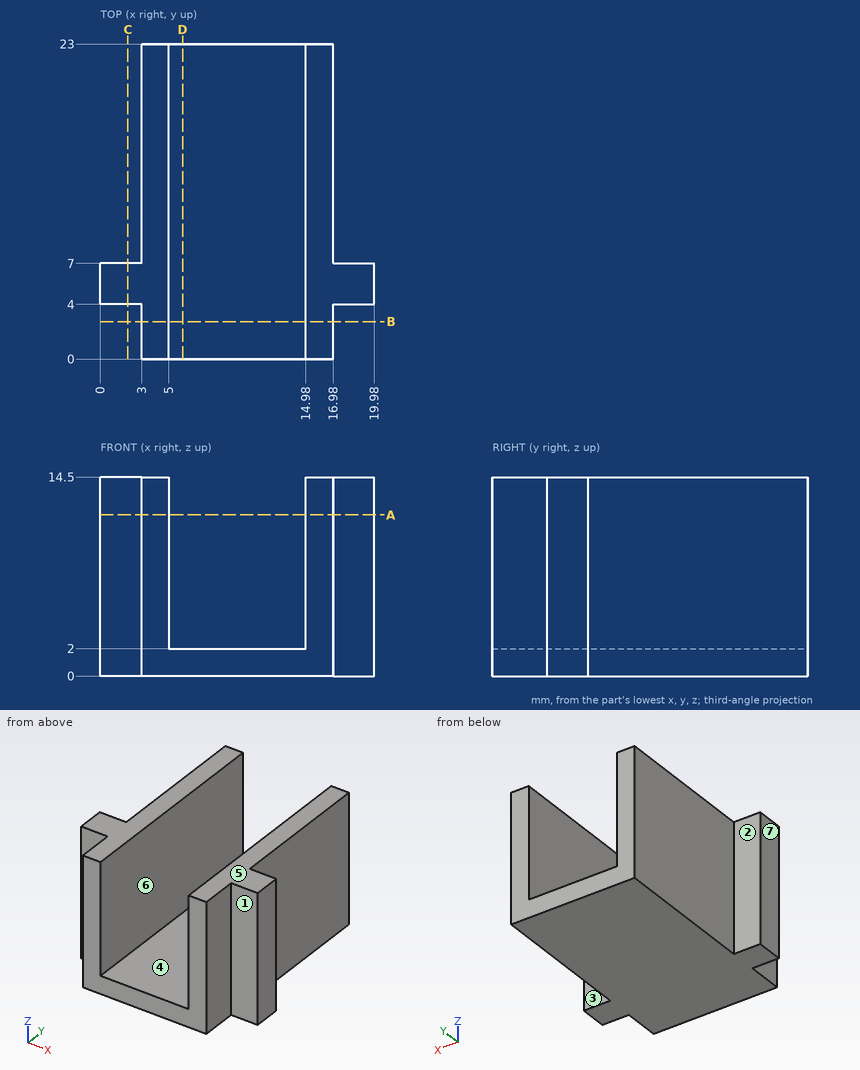
The drawing under review shows one solid part. Ordinate dimensions are in mm from its lowest x, y, z. A direction names the side the tool comes from. Coordinates: 2 decimals unless noted, no trailing zeros. Order: outer loops, then holes, each group sorted by start corner. A loop starts at its lowest first (then second) coordinate and runs counter-clockwise, first axis right, second up. Notation, with made-up numbers: (-4, 27) - (28, 27) arc R23 ccw to (28, 43) - close; hole circle Ø11 at (-34, 48.5). An arc over 180 degrees is marked (long way). Put each result on its own line as item: value.
1) Wall thickness on L1, parallel to X at y = 2.5, z = 9.25; L2, parallel to X at y = 5.5, z = 9; L3, parallel to Z at x = 11.25, y = 13.5: over which ranges is each line inside the solid? List them lowest first. Write a range as from..to.
Response values:
L1: x = 3..5, 14.98..16.98
L2: x = 0..5, 14.98..19.98
L3: z = 0..2
2) Take a section at A-A, the plane z = 11.75. Give the boundary of the cut face in (x, y).
Response values:
outline: (0, 4) - (3, 4) - (3, 0) - (5, 0) - (5, 23) - (3, 23) - (3, 7) - (0, 7) - close; (14.98, 0) - (16.98, 0) - (16.98, 4) - (19.98, 4) - (19.98, 7) - (16.98, 7) - (16.98, 23) - (14.98, 23) - close
3) Take a section at C-C, the plane x = 2. Give the boundary of the cut face in (y, z).
Response values:
outline: (4, 0) - (7, 0) - (7, 14.5) - (4, 14.5) - close
4) Take a section at B-B, the plane y = 2.75. Give the boundary of the cut face in (x, z).
Response values:
outline: (3, 0) - (16.98, 0) - (16.98, 14.5) - (14.98, 14.5) - (14.98, 2) - (5, 2) - (5, 14.5) - (3, 14.5) - close
5) Insertion check: P1, Ø4, axis at y = 11, z = 8.5, coming from the -X side; P2, Ø2.5, axis at x = 1.5, z = 10, coming from the -Y side; P3, Ø2, axis at y = 1.5, z = 4.5, coming from the +X side. Each pin has a flat end and moves straight along its axis. Give the tip position at first contact, or say it passes through.
Response values:
P1: stops at x = 3
P2: stops at y = 4
P3: stops at x = 16.98
6) Take a section at D-D, the plane x = 6. Give the boundary of the cut face in (y, z).
Response values:
outline: (0, 0) - (23, 0) - (23, 2) - (0, 2) - close
7) The part is to be moulded in two halves that separate along X. For the marked faces 5, 6 and 7, say which applies: released by +X, released by -X, zero draft, split by the parting line, or undercut.
Response values:
face 5: zero draft
face 6: undercut
face 7: released by -X
8) Tool access review of the marked faces 1, 2, 3 and 4: name each direction out of +Z, -Z, +X, -X, +Y, -Y from which nothing blocks a thin tool from reaching the whole face with its end or side.
Response values:
face 1: +Z, -Z, +X, -Y
face 2: +Z, -Z, -X, +Y
face 3: +Z, -Z, +X, +Y
face 4: +Z, +Y, -Y
